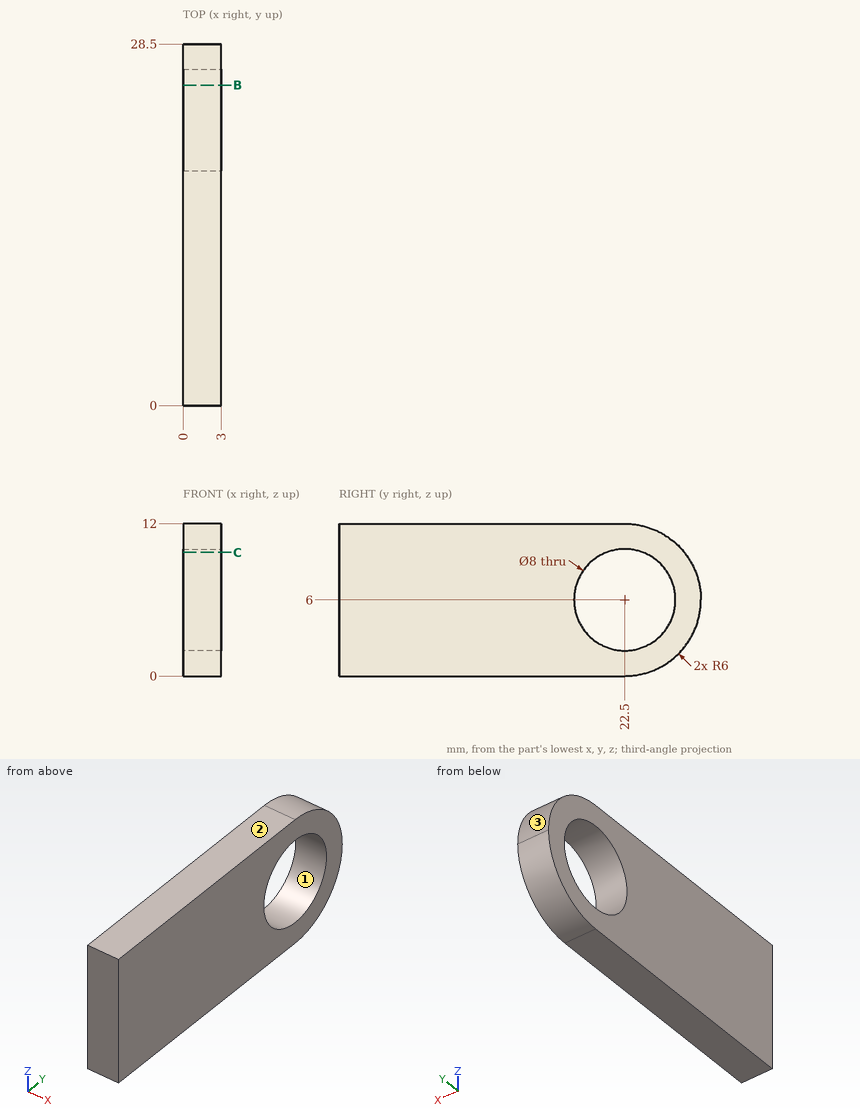
Job drawing, mm, ordinate dimensions from the low corner. One solid piece. Give positions to 0.01 mm unless a question says otherwise; leave off trailing zeros. Loops run counter-clockwise (first coordinate to the right, second up) from the corner with the lowest first, then second, coordinate; pieces in that order, holes last. Notation, with made-up numbers: M -8,80.25 L 22,80.25 A22 cw 22,111.25 Z; hole C 53.5,46.5 d8. An arc over 180 degrees is marked long. Return JSON: item names as keys, results as strings.
1) Pull direction Y, two halves, no side cores. Call the marked faces 1, 2 and 3: released by +Y, released by -Y, zero draft, split by the parting line, or undercut.
Calculated:
{"face 1": "undercut", "face 2": "zero draft", "face 3": "released by +Y"}
2) Saw through at B-B, the plane y = 25.25. List the corners of the cut face in (x, z) (1 decimal).
Calculated:
{"outline": "M 0,0.7 L 3,0.7 L 3,3.1 L 0,3.1 Z; M 0,8.9 L 3,8.9 L 3,11.3 L 0,11.3 Z"}
3) Flat gauge pin, fed straight in: pin 1 Ø1 at (x, z) = (2.5, 10.5) entering from -Y. Where does the tip first touch, or does it go through?
Calculated:
{"pin 1": "stops at y = 0"}
4) Drill centre lines: line 1 (Y direction, x = 0.65, z = 6); line 2 (Z direction, x = 2.35, y = 20.25) (1 decimal); line 3 (Y direction, x = 0.85, z = 7.75) (1 decimal). Where is each one in solid material? Low to high.
Calculated:
{"line 1": "y = 0 to 18.5, 26.5 to 28.5", "line 2": "z = 0 to 2.7, 9.3 to 12", "line 3": "y = 0 to 18.9, 26.1 to 28.2"}
5) Saw through at C-C, the plane z = 9.75. List the corners of the cut face in (x, y) (1 decimal).
Calculated:
{"outline": "M 0,0 L 3,0 L 3,21.1 L 0,21.1 Z; M 0,23.9 L 3,23.9 L 3,27.2 L 0,27.2 Z"}
